Autodesk Inventor part; units mm, degrees
ref_plane "YZ Plane" through (0, 0, 0) normal (1, 0, 0) x (0, 1, 0)
ref_plane "XZ Plane" through (0, 0, 0) normal (0, 1, 0) x (-1, 0, 0)
ref_plane "XY Plane" through (0, 0, 0) normal (0, 0, 1) x (1, 0, 0)
sketch "Sketch1" plane through (0, 0, 0) normal (0, 1, 0) x (-1, 0, 0)
  line L0 (46, 0) -> (-35, 0) construction
  line L1 (0, 54.3949) -> (0, -60) construction
  line L2 (17, -28) -> (17, 28)
  circle A0 centre (13.5, -18.75) radius 1.5
  line L3 (-17, 28) -> (-17, -28)
  line L4 (17, -28) -> (-17, -28)
  line L5 (17, 28) -> (33.782, 48)
  line L6 (17, 28) -> (43.1081, 28) construction
  line L7 (-17, 28) -> (-33.782, 48)
  arc A1 (33.782, 48) -> (-33.782, 48) centre (0, -24.5174) ccw
  line L8 (20, 48) -> (-20, 48)
  line L9 (-20, 48) -> (-20, 45)
  line L10 (-20, 45) -> (20, 45)
  line L11 (20, 45) -> (20, 48)
  circle A2 centre (0, 35) radius 1.5
  circle A3 centre (-13.5, -18.75) radius 1.5
  circle A4 centre (0, -10) radius 1.625
  line L12 (10, 31) -> (-10, 31)
  line L13 (-10, 31) -> (-10, 28)
  line L14 (-10, 28) -> (10, 28)
  line L15 (10, 28) -> (10, 31)
  point P0 (0, 0)
  dimension "d16" = 3
  dimension "d35" = 50
  dimension "d36" = 20
  dimension "d37" = 56
  dimension "d38" = 80
  dimension "d39" = 40
  dimension "d41" = 3
  dimension "d43" = 9.25
  dimension "d44" = 3
  dimension "d45" = 10
  dimension "d49" = 45
  dimension "d50" = 34
  dimension "d51" = 28
  dimension "d52" = 13.5
  dimension "d53" = 3.25
  dimension "d54" = 18
  dimension "d58" = 20
  dimension "d59" = 28
  dimension "d60" = 3
extrude "Extrusion3" add sketch "Sketch1" along normal blind 3 contours L4 L3 L7 A1 L5 L2 | L15 L14 L13 L12
fillet "Fillet3" radius 2 6 edges at (-33.782, 1.5, 48) (-17, 1.5, 28) (33.782, 1.5, 48) (17, 1.5, 28) (-17, 1.5, -28) (17, 1.5, -28)
extrude "Extrusion4" cut sketch "Sketch1" along normal blind 3 contours L15 L14 L13 L12
properties part number "bracket_camera_bottom"
CAD build for the part. Positions are in the model's coordinates, mm. A direction names the side the tool comes from. Round coordinates to 2 decimals unless told otherwise and drop trailing zeros. Write each loop counter-clockwise with the first axis right and the second up, starting at its lowest first coordinate (ties: lowest second). Pieces come first, ordered by that corner, then holes. Notation, with made-up numbers: (-8.5, 12) -> (3.5, 12) arc R5 ccw to (3.5, 20) -> close; hole circle Ø2 at (70.25, 84.5). An arc over 180 degrees is marked (long way). Answer in a Markdown table with one row per item. Add a question column.
Item 1: Saw through at A-A, the plane x = 0. Write the cut outline in (y, z) (3 decimals).
Item 2: Saw through at B-B, the plane z = -18.75. Write the cut outline in (x, y), then the cut area to 3 significant figures.
Item 3: Saw through at C-C, the plane y = 2.3. Write the cut outline in (x, z) (3 decimals).
Item 4: Mould opens along X. For faces 4 (the face through (0, 3, 14)), 5 (the face through (-32.495, 1.521, 47.694)), 6 (the face through (16.43, 1.52, -27.4)), 7 (the face through (20, 1, 47)) say: pulls with the +X half, pulls with the -X half, needs draft (parallel to the pull), parting line crosses it, or undercut.
Item 5: Drill centre lines: line 1 (Z direction, x = 0, y = 0.9) (3 decimals); line 2 (Z direction, x = -3, y = 0.3); line 3 (Z direction, x = 13.5, y = 2.15). Where is each one in solid material? Low to high. Write a range as from..to.
Item 6: Drop flat-ended pins along their axis: pin 1 Ø0.9 at (x, y) = (9.5, 1.5) entering from +Z; pin 2 Ø1.5 at (y, z) = (1, -3) entering from -X; pin 3 Ø1.5 at (x, y) = (19, 1) entering from -Z. Give the stop position or say it passes through.
Item 7: Which spindle directions (+Z, -Z, +X, -X, +Y, -Y) get a long thin tool onto all of the face, cutting with end or side? Do faces 1 (the face through (-10, 1, 29)), 2 (the face through (17, 1, 1)), 3 (the face through (-16.4, 1.52, -27.43)). Say none if no direction does.
Item 8: Saw through at D-D, the plane x = -19. Write the cut outline in (y, z).
Findings below:
| question | item | result |
|---|---|---|
| 1 | outline | (0, -28) -> (3, -28) -> (3, -11.625) -> (0, -11.625) -> close; (0, -8.375) -> (3, -8.375) -> (3, 28) -> (0, 28) -> close; (0, 31) -> (3, 31) -> (3, 33.5) -> (0, 33.5) -> close; (0, 36.5) -> (3, 36.5) -> (3, 45) -> (0, 45) -> close; (0, 48) -> (3, 48) -> (3, 55.483) -> (0, 55.483) -> close |
| 2 | outline | (-17, 0) -> (-15, 0) -> (-15, 3) -> (-17, 3) -> close; (-12, 0) -> (12, 0) -> (12, 3) -> (-12, 3) -> close; (15, 0) -> (17, 0) -> (17, 3) -> (15, 3) -> close |
| 2 | area | 84.0 mm^2 |
| 3 | outline | (-32.077, 45.968) -> (-17.468, 28.558) arc R2 cw to (-17, 27.272) -> (-17, -26) arc R2 ccw to (-15, -28) -> (15, -28) arc R2 ccw to (17, -26) -> (17, 27.272) arc R2 cw to (17.468, 28.558) -> (32.077, 45.968) arc R2 ccw to (31.328, 49.094) arc R80 ccw to (-31.328, 49.094) arc R2 ccw to start; hole (-20, 45) -> (20, 45) -> (20, 48) -> (-20, 48) -> close; hole circle Ø3 at (-13.5, -18.75); hole (-10, 28) -> (10, 28) -> (10, 31) -> (-10, 31) -> close; hole circle Ø3.25 at (0, -10); hole circle Ø3 at (0, 35); hole circle Ø3 at (13.5, -18.75) |
| 4 | face 4 | needs draft |
| 4 | face 5 | pulls with the -X half |
| 4 | face 6 | pulls with the +X half |
| 4 | face 7 | undercut |
| 5 | line 1 | z = -28..-11.625, -8.375..28, 31..33.5, 36.5..45, 48..55.483 |
| 5 | line 2 | z = -28..28, 31..45, 48..55.43 |
| 5 | line 3 | z = -28..-20.25, -17.25..45, 48..54.34 |
| 6 | pin 1 | stops at z = 54.97 |
| 6 | pin 2 | stops at x = -17 |
| 6 | pin 3 | stops at z = 29.49 |
| 7 | face 1 | +Y, -Y |
| 7 | face 2 | -Z, +X, +Y, -Y |
| 7 | face 3 | -Z, -X, +Y, -Y |
| 8 | outline | (0, 30.38) -> (3, 30.38) -> (3, 45) -> (0, 45) -> close; (0, 48) -> (3, 48) -> (3, 53.19) -> (0, 53.19) -> close |
